Autodesk Inventor part; units mm, degrees
ref_plane "Start Plane" through (0, 0, 0) normal (0, 1, 0) x (-1, 0, 0)
ref_plane "End Plane" through (0, 100, 0) normal (0, 1, 0) x (-1, 0, 0)
ref_plane "YZ Plane" through (0, 0, 0) normal (1, 0, 0) x (0, 1, 0)
ref_plane "Start Plane" through (0, 0, 0) normal (0, 1, 0) x (-1, 0, 0)
ref_plane "End Plane" through (0, 100, 0) normal (0, 1, 0) x (-1, 0, 0)
sketch "Sketch1" plane through (0, 0, 0) normal (0, 1, 0) x (-1, 0, 0)
  arc A0 (-3.05, -5.5) -> (-3.05, -5.1) centre (-3.05, -5.3) ccw
  line L0 (-3.05, -5.1) -> (-3.1625, -5.1)
  line L1 (-3.1625, -5.1) -> (-3.1625, -0.2474)
  line L2 (-3.1625, -0.2474) -> (-2.95, -0.0349)
  line L3 (-2.95, -0.0349) -> (-2.95, 4.06)
  arc A1 (-2.55, 4.46) -> (-2.95, 4.06) centre (-2.55, 4.06) ccw
  line L4 (-2.55, 4.46) -> (-1.373, 4.46)
  arc A2 (-0.9732, 4.074) -> (-1.373, 4.46) centre (-1.373, 4.06) ccw
  line L5 (-0.9732, 4.074) -> (-0.775, -1.6018)
  arc A3 (0.775, -1.6018) -> (-0.775, -1.6018) centre (0, -4.5) ccw
  line L6 (0.775, -1.6018) -> (0.9732, 4.074)
  arc A4 (1.373, 4.46) -> (0.9732, 4.074) centre (1.373, 4.06) ccw
  line L7 (1.373, 4.46) -> (2.55, 4.46)
  arc A5 (2.95, 4.06) -> (2.55, 4.46) centre (2.55, 4.06) ccw
  line L8 (2.95, 4.06) -> (2.95, -0.0349)
  line L9 (2.95, -0.0349) -> (3.1625, -0.2474)
  line L10 (3.1625, -0.2474) -> (3.1625, -5.1)
  line L11 (3.1625, -5.1) -> (3.05, -5.1)
  arc A6 (3.05, -5.1) -> (3.05, -5.5) centre (3.05, -5.3) ccw
  line L12 (3.05, -5.5) -> (6.5, -5.5)
  line L13 (6.5, -5.5) -> (6.5, -4.5)
  line L14 (6.5, -4.5) -> (5.2125, -4.5)
  arc A7 (4.2125, -3.5) -> (5.2125, -4.5) centre (5.2125, -3.5) ccw
  line L15 (4.2125, -3.5) -> (4.2125, 0.1875)
  line L16 (4.2125, 0.1875) -> (4, 0.4)
  line L17 (4, 0.4) -> (4, 4.4)
  arc A8 (4, 4.4) -> (2.9, 5.5) centre (2.9, 4.4) ccw
  line L18 (2.9, 5.5) -> (-2.9, 5.5)
  arc A9 (-2.9, 5.5) -> (-4, 4.4) centre (-2.9, 4.4) ccw
  line L19 (-4, 4.4) -> (-4, 0.4)
  line L20 (-4, 0.4) -> (-4.2125, 0.1875)
  line L21 (-4.2125, 0.1875) -> (-4.2125, -3.5)
  arc A10 (-5.2125, -4.5) -> (-4.2125, -3.5) centre (-5.2125, -3.5) ccw
  line L22 (-5.2125, -4.5) -> (-6.5, -4.5)
  line L23 (-6.5, -4.5) -> (-6.5, -5.5)
  line L24 (-6.5, -5.5) -> (-3.05, -5.5)
  point P0 (0, 0)
extrude "Body" add sketch "Sketch1" along normal up to surface (100 mm away) from surface at 0
sketch "Sketch2" plane through (0, 0, 0) normal (0, 1, 0) x (-1, 0, 0)
  line L0 (0, 0) -> (10, 0)
ref_plane "Work Plane3" through (0, 0, 0) normal (0, 0, -1) x (-1, 0, 0)
sketch "Sketch3" plane through (0, 0, 0) normal (0, 0, -1) x (-1, 0, 0)
  line L0 (-9.8, 0) -> (13.3, 0)
  line L1 (-9.8, 100) -> (13.3, 100)
  dimension "d7" = 100
equation "\"G_OFFSET_START\" = 0"
equation "\"G_OFFSET_END\" = 0"
equation "\"G_L\" = d7"
properties part number "13-106"
Read the model definition and answer for the solid it produces. Units are mm, in the model's axes. A direction names the side the tool comes from. Give positions to 0.01 mm unless a question says otherwise; leave off trailing zeros.
(1) Given pin 1 (1.3 mm diameter, centred on x = -2, y = 68, fed in from -Z); pin 2 (3.5 mm diameter, centred on y = 50, z = 3, fed in from -X); pin 3 (1.4 mm diameter, centred on x = -6, y = 60.5, fed in from +Z), each flat-ended and moving along its own axis, determine where each tip first touches the part or whether it passes through.
(2) Straight lines are drawn through the part: L1, parallel to X at y = 90, z = 3.75; L2, parallel to X at y = 74, z = -3.25; L3, parallel to X at y = 59, z = 2. For each, find the intervals that lie inside material, in ascending order.
(3) For a pull along X with two mould halves and no side action, classify faces 1 (the flat face through (-3.162, 49, -3)), 2 (the cylindrical face through (0, 49.3, -1.5)), 3 (the flat face through (0, 100, 0)), 4 (the flat face through (4.212, 49, -2)) as released by +X, released by -X, zero draft, split by the parting line, or undercut.
(4) For faces 5 (the flat face through (-4.212, 49, -2)), 6 (the flat face through (5, 49, -5.5)), 7 (the flat face through (4, 49, 2)), 8 (the flat face through (-2.95, 49, 2)), determine the directions among +Z, -Z, +X, -X, +Y, -Y from which every point of the face is accessible in a straight line to the end or side of a thin tool.
Result sheet:
1. pin 1: stops at z = 4.45
1. pin 2: stops at x = -4
1. pin 3: stops at z = -4.5
2. L1: x = -4 to -2.95, -0.96 to 0.96, 2.95 to 4
2. L2: x = -4.21 to -3.16, 3.16 to 4.21
2. L3: x = -4 to -2.95, -0.9 to 0.9, 2.95 to 4
3. face 1: undercut
3. face 2: undercut
3. face 3: zero draft
3. face 4: released by +X
4. face 5: +Z, -X, +Y, -Y
4. face 6: -Z, +X, -X, +Y, -Y
4. face 7: +Z, +X, +Y, -Y
4. face 8: +Y, -Y
